```python
from build123d import *

# Parameters (mm, degrees)
F0_R     = 10
F1_DEPTH = 10


with BuildPart() as f1:
    # F0 (on Top) → F1 (new body)
    with BuildSketch(Plane.XY):
        Polygon((-80, 0), (-80, -79.253925), (80, -79.253925), (80, 0.746075), (64.365849, 68.231762), (0, 95.746075), (-64.365849, 68.231762), align=None)
        Circle(F0_R, mode=Mode.SUBTRACT)
    extrude(amount=F1_DEPTH)


solid = f1.part
```
Design review of the part built by this model. Coordinates are the model's own, in mm. Give positions to 0.01 mm unless a question says otherwise; leave off trailing zeros. Write each loop counter-clockwise with the first axis right and the second up, starting at its lowest first coordinate (ties: lowest second). Pieces come first, ordered by that corner, then holes. Notation, with made-up numbers: (34.5, 5) -> (65.5, 5) arc R19 cw to (65.5, 16) -> close; hole circle Ø1 at (-13.75, -29). An arc over 180 degrees is marked (long way). Answer in a Markdown table with one row per item.
(1) Consider section C-C (y = 24). State the section outline as (x, z) points.
Results:
| item | result |
|---|---|
| outline | (-74.5, 0) -> (74.61, 0) -> (74.61, 10) -> (-74.5, 10) -> close |
(2) Clearance check with flat-ended pins moving along their axes: pin 1 (3 mm diameter, centred on y = 66.5, z = 5.5, fed in from -X); pin 2 (1 mm diameter, centred on x = 13.5, z = 2.5, fed in from +Y); pin 3 (4 mm diameter, centred on y = 12, z = 1, fed in from +X). State where each tip first meets the part, or that it passes through.
Results:
| item | result |
|---|---|
| pin 1 | x = -65.11 |
| pin 2 | y = 90.19 |
| pin 3 | x = 77.86 |
(3) To check wall thickness, follow probe 1 along Y at (x, z) = (0, 5.5); probe 2 along X at (y, z) = (-4.5, 6.5); probe 3 along Y at (x, z) = (-17, 7.5). State the ranges of each line that lie inside material, in increasing order.
Results:
| item | result |
|---|---|
| probe 1 | -79.25 to -10, 10 to 95.75 |
| probe 2 | -80 to -8.93, 8.93 to 80 |
| probe 3 | -79.25 to 88.48 |
(4) Mouldability with a two-part tool opening along Y and no side actions: class faces 1 (the flat face through (-19, 9, 10)), 2 (the flat face through (-72.073, 34.594, 4.93)), 3 (the cylindrical face through (-2.17, -9.76, 4.93)) as +Y half, -Y half, draft (parallel to the pull), parting line (faces both ways), or undercut.
Results:
| item | result |
|---|---|
| face 1 | draft |
| face 2 | +Y half |
| face 3 | undercut |
(5) Consider section A-A (z = 7). State the section outline as (x, y) points, then the cut area to 3 significant figures.
Results:
| item | result |
|---|---|
| outline | (-80, -79.25) -> (80, -79.25) -> (80, 0.75) -> (64.37, 68.23) -> (0, 95.75) -> (-64.37, 68.23) -> (-80, 0) -> close; hole circle Ø20 at (0, 0) |
| area | 24,000 mm2 |
(6) Consider section B-B (x = 32.5). State the section outline as (y, z) points, then the cut area to 3 significant figures.
Results:
| item | result |
|---|---|
| outline | (-79.25, 0) -> (81.85, 0) -> (81.85, 10) -> (-79.25, 10) -> close |
| area | 1,610 mm2 |
